Source: CAD feature listing. Evaluate the final solid. Frame: model axes, mm. Round coordinates to 2 decimals unless told otherwise and drop trailing zeros. Write each loop counter-clockwise with the first axis right and the second up, starting at its lowest first coordinate (ties: lowest second). Pieces come first, ordered by that corner, then holes. Notation, with made-up numbers: M 49.25,-3 L 106.25,-3 A18 cw 106.25,26 Z; hole C 68.25,-28 d6. An arc over 180 degrees is marked long. Answer in a Markdown table with one row per item. Add a question column.
Item 1: Material intervals for probe 1 along Z at (x, y) = (0, 1.5); probe 2 along X at (y, z) = (4.45, 132.5); probe 3 along Z at (x, y) = (3, 4.3), sorted ascending.
Item 2: Cut plane B-B on y = 4.65. Return loops of the section in (x, z).
Item 3: Mould query, pull axis X, two halves, no side actions, for faces 1 (the face through (-1.302, 2.958, 122.585)), 2 (the face through (-17.5, 3, -2)), 3 (the face through (5.38, 2.96, -140.93)), 4 (the face through (0, 3, -150)). Classes: released by +X, released by -X, zero draft, split by the parting line, or undercut.
Item 4: Contact query for flat-ended pins moving along their axis: pin 1 (2 mm diameter, centred on x = 3, y = 2.5, fed in from -Z); pin 2 (1.5 mm diameter, centred on x = -6.5, y = 1.5, fed in from +Z); pin 3 (1 mm diameter, centred on x = 8, y = 3, fed in from +Z). Output: stop coordinate, or through.
Item 5: Cut plane A-A on x = 0. Return loops of the section in (y, z), and give its area (3 significant figures).
from build123d import *

# Parameters (mm, degrees)
SKETCH1_R           = 17.5
SKETCH1_R_2         = 10
BOSS_EXTRUDE1_DEPTH = 6


with BuildPart() as part:
    # Sketch1 → Boss-Extrude1 (new body)
    with BuildSketch(Plane(origin=(0, 0, 0), x_dir=(1, 0, 0), z_dir=(0, 1, 0))):
        with BuildLine():
            ThreePointArc((17.5, 132.5), (0, 115), (-17.5, 132.5))
            Line((-17.5, 132.5), (-17.5, -132.5))
            ThreePointArc((-17.5, -132.5), (0, -115), (17.5, -132.5))
            Line((17.5, -132.5), (17.5, 132.5))
        make_face()
        with Locations((0, 132.5)):
            Circle(SKETCH1_R)
        with Locations((0, 132.5)):
            Circle(SKETCH1_R_2, mode=Mode.SUBTRACT)
        with Locations((0, -132.5)):
            Circle(SKETCH1_R)
        with Locations((0, -132.5)):
            Circle(SKETCH1_R_2, mode=Mode.SUBTRACT)
    extrude(amount=BOSS_EXTRUDE1_DEPTH)


solid = part.part
Results below:
| question | item | result |
|---|---|---|
| 1 | probe 1 | -150 to -142.5, -122.5 to 122.5, 142.5 to 150 |
| 1 | probe 2 | -17.5 to -10, 10 to 17.5 |
| 1 | probe 3 | -149.74 to -142.04, -122.96 to 122.96, 142.04 to 149.74 |
| 2 | outline | M -17.5,-132.5 A17.5 ccw 17.5,-132.5 L 17.5,132.5 A17.5 ccw -17.5,132.5 Z; hole C 0,-132.5 d20; hole C 0,132.5 d20 |
| 3 | face 1 | undercut |
| 3 | face 2 | released by -X |
| 3 | face 3 | undercut |
| 3 | face 4 | split by the parting line |
| 4 | pin 1 | z = -149.89 |
| 4 | pin 2 | z = 149.03 |
| 4 | pin 3 | z = 148.31 |
| 5 | outline | M 0,-150 L 6,-150 L 6,-142.5 L 0,-142.5 Z; M 0,-122.5 L 6,-122.5 L 6,122.5 L 0,122.5 Z; M 0,142.5 L 6,142.5 L 6,150 L 0,150 Z |
| 5 | area | 1,560 mm2 |
